Autodesk Inventor part; units mm, degrees
ref_plane "to_bolt_XY" through (5, -8, 0) normal (1, 0, 0) x (0, 0, -1)
ref_plane "to_bolt_YZ" through (5, -8, 0) normal (0, 0, -1) x (0, 1, 0)
ref_plane "to_bolt_ZX" through (5, -8, 0) normal (0, 1, 0) x (1, 0, 0)
sketch "Sketch_14" plane through (0, 0, 0) normal (1, 0, 0) x (0, 1, 0)
  line L0 (0, -4) -> (0, 4)
  line L1 (0, 4) -> (12, 4)
  line L2 (12, 4) -> (12.5, 3.5)
  line L3 (12.5, 3.5) -> (12.5, -3.5)
  line L4 (12.5, -3.5) -> (12, -4)
  line L5 (12, -4) -> (0, -4)
  line L6 (0, -4) -> (0, 4)
revolve "Revolution1" add sketch "Sketch_14" angle 360 about axis through (0, 0, -4) along (0, 0, -1)
sketch "Sketch_15" plane through (0, 0, 0) normal (1, 0, 0) x (0, 1, 0)
  line L0 (0, -4) -> (0, 4)
  line L1 (0, 4) -> (4.5, 4)
  line L2 (4.5, 4) -> (4, 3.5)
  line L3 (4, 3.5) -> (4, -3.5)
  line L4 (4, -3.5) -> (4.5, -4)
  line L5 (4.5, -4) -> (0, -4)
  line L6 (0, -4) -> (0, 4)
revolve "Revolution2" cut sketch "Sketch_15" angle 360 about axis through (0, 0, -4) along (0, 0, -1)
sketch "Sketch_16" plane through (0, 0, 0) normal (0, 0, 1) x (1, 0, 0)
  arc A0 (-0.75, -13.4792) -> (0.75, -13.4792) centre (0, 0) ccw
  line L0 (0.75, -13.4792) -> (0.75, 0)
  line L1 (0.75, 0) -> (-0.75, 0)
  line L2 (-0.75, 0) -> (-0.75, -13.4792)
extrude "Extrusion1" cut sketch "Sketch_16" along normal mid plane 8
sketch "Sketch4" plane through (0, 0, -4) normal (0, 0, -1) x (-1, 0, 0)
  point P0 (-7, 0)
hole "Hole1" at (7, 0, -4) direction (0, 0, 1) diameter 3.5 depth 8
sketch "Sketch5" plane through (0, 0, -4) normal (0, 0, -1) x (-1, 0, 0)
  point P0 (7, 0)
hole "Hole2" at (-7, 0, -4) direction (0, 0, 1) diameter 3.5 depth 8
sketch "Sketch6" plane through (0, 0, -4) normal (0, 0, -1) x (-1, 0, 0)
  point P0 (0, 7)
hole "Hole3" at (0, 7, -4) direction (0, 0, 1) diameter 3.5 depth 8
sketch "Sketch_23" plane through (0, -8, 0) normal (0, 1, 0) x (1, 0, 0)
  line L0 (12.5, 0) -> (0, 0)
  line L1 (0, 0) -> (0, 1.7)
  line L2 (0, 1.7) -> (5, 1.7)
  line L3 (5, 1.7) -> (5, 3)
  line L4 (5, 3) -> (12.5, 3)
  line L5 (12.5, 3) -> (12.5, 0)
  line L6 (12.5, 0) -> (0, 0)
revolve "Revolution3" cut sketch "Sketch_23" angle 360 about axis through (12.5, -8, 0) along (1, 0, 0)
sketch "Sketch8" plane through (-0.75, -11.9765, 4) normal (1, 0, 0) x (0, 0, -1)
  point P0 (4, 3.9765)
hole "Hole4" at (-0.75, -8, 0) direction (-1, 0, 0) diameter 2.459 depth 9.9271 countersink diameter 3 countersink angle 90
ref_plane "to_bolt_XY" through (5, -8, 0) normal (1, 0, 0) x (0, 0, -1)
ref_plane "to_bolt_YZ" through (5, -8, 0) normal (0, 0, -1) x (0, 1, 0)
ref_plane "to_bolt_ZX" through (5, -8, 0) normal (0, 1, 0) x (1, 0, 0)
properties part number "SCST8-8b"
Here's how the part is built. I have some questions about the finished solid (model axes, mm). A direction names the side the tool comes from. Round coordinates to 2 decimals unless told otherwise and drop trailing zeros. Write each loop counter-clockwise with the first axis right and the second up, starting at its lowest first coordinate (ties: lowest second). Pieces come first, ordered by that corner, then holes.
1. I need wall thicknesses on L1, parallel to X at y = 0, z = -1.25; L2, parallel to Y at x = 0, z = -1.25; L3, parallel to X at y = -1.25, z = 1.75. Which ranges of each line are inside material? Lowest first, please.
2. Suppose I cut it at C-C (x = -7). State how many separate pieces and enclosed holes the cut face has, and give its area (3 significant figures).
3. Suppose I cut it at A-A (y = 0). List the corners of the cut face in (x, z) for me, and give its area (3 significant figures).
4. For faces 1 (the flat face through (5, -10, 0)), 2 (the cylindrical face through (-5.29, -0.38, 0.06)), 3 (the flat face through (-0.75, -8, -2)), which set-ups out of +Z, -Z, +X, -X, +Y, -Y let a thin tool reach every point of the face, with its end or its side?
5. Suppose I cut it at B-B (z = 0). List the corners of the cut face in (x, y) for me, and give its area (3 significant figures).
6. Will these pins go through, and if not, where does the flat tip stop? pin 1 Ø4 at (x, z) = (-3.5, -1) entering from +Y; pin 2 Ø2 at (y, z) = (-9, 2.5) entering from +X; pin 3 Ø3 at (x, z) = (10, -3) entering from -Y; pin 4 Ø5.5 at (x, y) = (7, 0) entering from +Z.
7. If we mould it in two halves opening along Y, with no side actions, what happens to faces 4 (the cylindrical face through (2.9, -9.66, 0.37)), 5 (the conical face through (-0.52, 12.13, 3.86)), 6 (the flat face through (0.75, -8, -2))? For each: released by +Y, released by -Y, zero draft, split by the parting line, or undercut.
Answer sheet:
1. L1: x = -12.5 to -8.75, -5.25 to -4, 4 to 5.25, 8.75 to 12.5
1. L2: y = 4 to 5.25, 8.75 to 12.5
1. L3: x = -12.44 to -8.22, -5.78 to -3.8, 3.8 to 5.78, 8.22 to 12.44
2. separate pieces: 2
2. enclosed holes: 1
2. area: 132 mm2
3. outline: (-12.5, -3.5) - (-12, -4) - (-8.75, -4) - (-8.75, 4) - (-12, 4) - (-12.5, 3.5) - close; (-5.25, -4) - (-4.5, -4) - (-4, -3.5) - (-4, 3.5) - (-4.5, 4) - (-5.25, 4) - close; (4, -3.5) - (4.5, -4) - (5.25, -4) - (5.25, 4) - (4.5, 4) - (4, 3.5) - close; (8.75, -4) - (12, -4) - (12.5, -3.5) - (12.5, 3.5) - (12, 4) - (8.75, 4) - close
3. area: 79.0 mm2
4. face 1: +X
4. face 2: +Z, -Z
4. face 3: +Z, -Z, -Y
5. outline: (-10.51, -6.77) - (-1.02, -6.77) - (-0.75, -6.5) - (-0.75, -3.93) arc R4 cw (long way) to (0.75, -3.93) - (0.75, -6.3) - (5, -6.3) - (5, -5) - (11.46, -5) arc R12.5 ccw (long way) to start; (-8.43, -9.23) arc R12.5 ccw to (-0.75, -12.48) - (-0.75, -9.5) - (-1.02, -9.23) - close; (0.75, -12.48) arc R12.5 ccw to (5.94, -11) - (5, -11) - (5, -9.7) - (0.75, -9.7) - close; hole circle Ø3.5 at (-7, 0); hole circle Ø3.5 at (0, 7); hole circle Ø3.5 at (7, 0)
5. area: 337 mm2
6. pin 1: stops at y = 12.41
6. pin 2: stops at x = 9.49
6. pin 3: stops at y = -9.17
6. pin 4: stops at z = 4
7. face 4: undercut
7. face 5: split by the parting line
7. face 6: zero draft
